Part model, mm, in its own coordinate system. A direction names the side the tool comes from. Round coordinates to 2 decimals unless told otherwise and drop trailing zeros. Loops run counter-clockwise (first coordinate to the right, second up) from the corner with the lowest first, then second, coordinate; pieces in that order, holes last. Notation, with made-up numbers: M 66.25,61.25 L 109.25,61.25 A7 cw 109.25,73.25 Z; hole C -28.75,48 d5. An arc over 180 degrees is marked long. Put each result on its own line as item: value. Start each with the question number.
1) Slice it at C-C on x = -24. Give the cut face in (y, z).
2) Which spindle directions (+Z, -Z, +X, -X, +Y, -Y) get a long thin tool onto all of the face, cutting with end or side? Do faces 4 (the flat face through (3, 7, 0)), 5 (the flat face through (-14.962, 33, 25)), 6 (the flat face through (-12, 30.257, 25)). Say none if no direction does.
3) Slice it at A-A on x = -11. Give the cut face in (y, z), then the cut area to 3 significant figures.
4) Pull direction Y, two halves, no side cores. Call faces 1 (the flat face through (-28.962, 33, 25)), 2 (the flat face through (-33, 36.242, 25)), 3 (the flat face through (-34.462, 25, 25)): +Y half, -Y half, draft (parallel to the pull), parting line (faces both ways), or undercut.
5) Probe line 1 along Y through (x, z) = (-13.5, 21); line 2 along X through (y, z) = (23.5, 39.5); line 3 along Y through (x, z) = (-16.5, 6.5). List the from-to ranges inside material, lowest first.
6) Drop flat-ended pins along their axis: pin 1 Ø1.5 at (x, z) = (31, 17.5) entering from +Y; pin 2 Ø8 at (x, y) = (21.5, -10.5) entering from -Z. Give the stop position or say it passes through.
7) Slice it at B-B on z = 46.5. Give the cut face in (x, y).
Autodesk Inventor part; units mm, degrees
ref_plane "YZ Plane" through (0, 0, 0) normal (1, 0, 0) x (0, 1, 0)
ref_plane "XZ Plane" through (0, 0, 0) normal (0, 1, 0) x (-1, 0, 0)
ref_plane "XY Plane" through (0, 0, 0) normal (0, 0, 1) x (1, 0, 0)
sketch "Sketch1" plane through (0, 0, 0) normal (0, 0, 1) x (1, 0, 0)
  line L0 (-36.9152, 36.2425) -> (43.0848, 36.2425)
  line L1 (43.0848, 36.2425) -> (43.0848, -23.7575)
  line L2 (43.0848, -23.7575) -> (-36.9152, -23.7575)
  line L3 (-36.9152, -23.7575) -> (-36.9152, 36.2425)
  point P0 (0, 0)
  dimension "d0" = 80
  dimension "d1" = 60
extrude "Extrusion1" add sketch "Sketch1" along normal blind 50
sketch "Sketch2" plane through (0, 0, 50) normal (0, 0, 1) x (1, 0, 0)
  line L0 (-34.4619, 20.2567) -> (-34.4619, 30.2567)
  line L1 (-34.4619, 30.2567) -> (-28.9619, 30.2567)
  line L2 (-28.9619, 30.2567) -> (-28.9619, 39.2567)
  line L3 (-28.9619, 39.2567) -> (-14.9619, 39.2567)
  line L4 (-14.9619, 39.2567) -> (-14.9619, 30.2567)
  line L5 (-14.9619, 30.2567) -> (-9.4619, 30.2567)
  line L6 (-9.4619, 30.2567) -> (-9.4619, 20.2567)
  line L7 (-9.4619, 20.2567) -> (-34.4619, 20.2567)
  point P0 (0, 0)
  point P1 (-21.9619, 39.2567)
  dimension "d4" = 14
  dimension "d5" = 9
  dimension "d6" = 10
  dimension "d7" = 12.5
  dimension "d8" = 25
  dimension "d9" = 7
extrude "Extrusion2" cut sketch "Sketch2" against normal blind 50
sketch "Sketch5" plane through (0, 0, 50) normal (0, 0, 1) x (1, 0, 0)
  line L0 (31.2523, 36.3999) -> (38.2523, 36.3999)
  line L1 (38.2523, 36.3999) -> (38.2523, 32.8141)
  line L2 (38.2523, 32.8141) -> (39.6665, 31.3999)
  line L3 (39.6665, 31.3999) -> (38.2523, 29.9857)
  line L4 (38.2523, 29.9857) -> (36.8381, 31.3999)
  line L5 (36.8381, 31.3999) -> (31.2523, 31.3999)
  line L6 (31.2523, 36.3999) -> (31.2523, 31.3999) construction
  line L7 (31.2523, 36.3999) -> (24.2523, 36.3999)
  line L8 (24.2523, 36.3999) -> (24.2523, 32.8141)
  line L9 (24.2523, 32.8141) -> (22.8381, 31.3999)
  line L10 (22.8381, 31.3999) -> (24.2523, 29.9857)
  line L11 (24.2523, 29.9857) -> (25.6665, 31.3999)
  line L12 (25.6665, 31.3999) -> (31.2523, 31.3999)
  point P0 (0, 0)
  dimension "d27" = 7
  dimension "d28" = 2
  dimension "d29" = 2
  dimension "d30" = 135
  dimension "d31" = 90
  dimension "d32" = 5
  dimension "d33" = 2
extrude "Extrusion3" cut sketch "Sketch5" against normal blind 50
properties part number "PiesaSuportCanale"
Recorded:
1. outline: M -23.76,0 L 20.26,0 L 20.26,50 L -23.76,50 Z
2. face 4: -Z, +X, -X, +Y, -Y
2. face 5: +Z, -Z, +Y
2. face 6: +Z, -Z
3. outline: M -23.76,0 L 20.26,0 L 20.26,50 L -23.76,50 Z; M 30.26,0 L 36.24,0 L 36.24,50 L 30.26,50 Z
3. area: 2,500 mm2
4. face 1: draft
4. face 2: +Y half
4. face 3: undercut
5. line 1: y = -23.76 to 20.26, 30.26 to 36.24
5. line 2: x = -36.92 to -34.46, -9.46 to 43.08
5. line 3: y = -23.76 to 20.26
6. pin 1: stops at y = 31.4
6. pin 2: stops at z = 0
7. outline: M -36.92,-23.76 L 43.08,-23.76 L 43.08,36.24 L 38.25,36.24 L 38.25,32.81 L 39.67,31.4 L 38.25,29.99 L 36.84,31.4 L 25.67,31.4 L 24.25,29.99 L 22.84,31.4 L 24.25,32.81 L 24.25,36.24 L -14.96,36.24 L -14.96,30.26 L -9.46,30.26 L -9.46,20.26 L -34.46,20.26 L -34.46,30.26 L -28.96,30.26 L -28.96,36.24 L -36.92,36.24 Z
